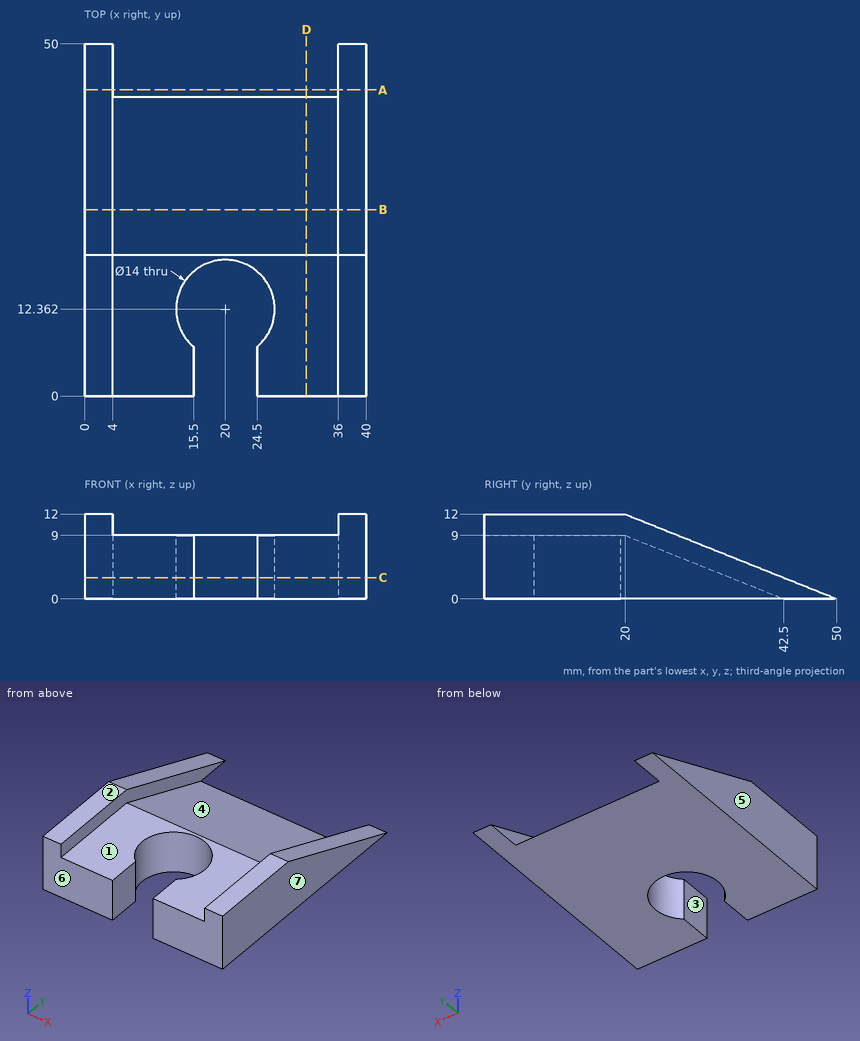
Source: three-view drawing plus pictorial views. Frame: mm from the lowest corner of the part. A direction names the side the tool comes from. Give positions to 0.01 mm unless a question says otherwise; leave off trailing zeros. Write each loop counter-clockwise with the first axis right and the second up, starting at its lowest first coordinate (ties: lowest second). Pieces come first, ordered by that corner, then holes. Notation, with made-up numbers: (26.25, 15) - (61.25, 15) arc R13 ccw to (61.25, 25) - close; hole circle Ø9 at (50, 61.25). An arc over 180 degrees is marked (long way). Write item = value, one per line. Start each with the question number.
Q1. Material intervals for probe 1 along X at (y, z) = (7.5, 11.75); probe 2 along Z at (x, y) = (15, 7); probe 3 along X at (y, z) = (8.5, 5.75), sorted ascending.
Q2. Cut plane C-C, the plane z = 3. Return loops of the section in (x, y), then the cut area to 3 significant figures.
Q3. Cut plane B-B, the plane y = 26.5. Return loops of the section in (x, z).
Q4. Cut plane A-A, the plane y = 43.5. Return loops of the section in (x, z).
Q5. Reachability of the marked faces 1, 2 and 3 from +Z, -Z, +X, -X, +Y, -Y: full face, straight path, thin tool, end or side. Return the list, or none.
Q6. Draft query along X for the marked faces 4, 5, 6 and 7. Return one class per face: +X half, -X half, draft (parallel to the pull), parting line (faces both ways), or undercut.
Q7. Cut plane D-D, the plane x = 31.5. Return loops of the section in (y, z), then the cut area to 3 significant figures.
Q8. Pin query (flat end, axial travel): pin 1 Ø6 at (x, y) = (24, 6.5) entering from +Z; pin 2 Ø4 at (x, z) = (19, 9) entering from -Y; pin 3 Ø1.5 at (x, z) = (7, 3) entering from +Y (1 decimal). Return the tip coordinate at first contact, or that it passes through.
Computed values:
q1.probe_1 = 0 to 4, 36 to 40
q1.probe_2 = 0 to 9
q1.probe_3 = 0 to 14.16, 25.84 to 40
q2.outline = (0, 0) - (15.5, 0) - (15.5, 7) arc R7 cw (long way) to (24.5, 7) - (24.5, 0) - (40, 0) - (40, 42.5) - (36, 42.5) - (36, 35) - (4, 35) - (4, 42.5) - (0, 42.5) - close
q2.area = 1,250 mm²
q3.outline = (0, 0) - (40, 0) - (40, 9.4) - (36, 9.4) - (36, 6.4) - (4, 6.4) - (4, 9.4) - (0, 9.4) - close
q4.outline = (0, 0) - (4, 0) - (4, 2.6) - (0, 2.6) - close; (36, 0) - (40, 0) - (40, 2.6) - (36, 2.6) - close
q5.face_1 = +Z, +Y, -Y
q5.face_2 = +Z, +X, -X, +Y, -Y
q5.face_3 = +Z, -Z, -Y
q6.face_4 = undercut
q6.face_5 = -X half
q6.face_6 = draft
q6.face_7 = +X half
q7.outline = (0, 0) - (42.5, 0) - (20, 9) - (0, 9) - close
q7.area = 281 mm²
q8.pin_1 = 9
q8.pin_2 = 18.69
q8.pin_3 = 36.9
